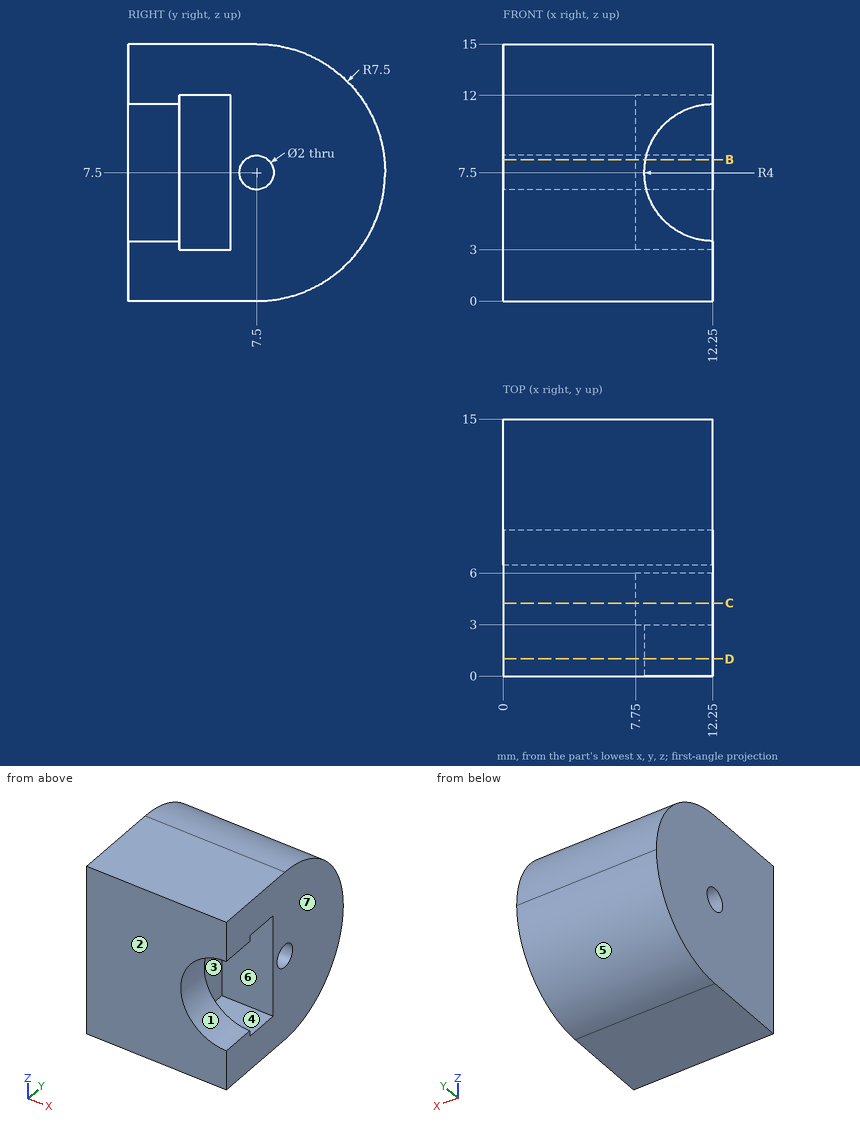
Can you work these out from the drawing? Everything is in mm from the part's minimum corner. A direction names the side the tool comes from. Coordinates: 2 decimals unless noted, no trailing zeros. Write each loop counter-clockwise with the first axis right and the second up, starting at its lowest first coordinate (ties: lowest second). Pieces come first, ordered by that corner, then holes. Notation, with made-up numbers: (-39.75, -25.75) -> (1.25, -25.75) arc R34 cw to (1.25, 13.25) -> close; hole circle Ø8 at (36, 0.5). An arc over 180 degrees is marked (long way). Return JSON: item names as keys, results as strings.
(1) Imagine slicing it at D-D, the plane y = 1. Please give me the cut outline in (x, z), then the cut area to 3 significant figures.
Numbers:
{"outline": "(0, 0) -> (12.25, 0) -> (12.25, 3.5) arc R4 cw to (12.25, 11.5) -> (12.25, 15) -> (0, 15) -> close", "area": "159 mm2"}
(2) We'd pull the mould along Y, two halves only. Please class the marked faces 4, 5, 6 and 7: +Y half, -Y half, draft (parallel to the pull), parting line (faces both ways), or undercut.
Numbers:
{"face 4": "undercut", "face 5": "+Y half", "face 6": "undercut", "face 7": "draft"}
(3) Imagine slicing it at C-C, the plane y = 4.25. Please give me the cut outline in (x, z), then the cut area to 3 significant figures.
Numbers:
{"outline": "(0, 0) -> (12.25, 0) -> (12.25, 3) -> (7.75, 3) -> (7.75, 12) -> (12.25, 12) -> (12.25, 15) -> (0, 15) -> close", "area": "143 mm2"}
(4) Imagine slicing it at B-B, the plane z = 8.25. Please give me the cut outline in (x, y), then the cut area to 3 significant figures.
Numbers:
{"outline": "(0, 0) -> (8.32, 0) -> (8.32, 3) -> (7.75, 3) -> (7.75, 6) -> (12.25, 6) -> (12.25, 6.84) -> (0, 6.84) -> close; (0, 8.16) -> (12.25, 8.16) -> (12.25, 14.96) -> (0, 14.96) -> close", "area": "142 mm2"}
(5) I'm going to push flat-ended pins straight in: pin 1 (3.5 mm diameter, centred on x = 9.5, z = 7, fed in from +Y); pin 2 (1.6 mm diameter, centred on y = 7.5, z = 7.5, fed in from +X); pin 3 (0.9 mm diameter, centred on y = 4.5, z = 6.5, fed in from +X); pin 4 (1.4 mm diameter, centred on x = 9.5, z = 8, fed in from -Y). Where does each tip first touch, or does it pass through?
Numbers:
{"pin 1": "stops at y = 15", "pin 2": "passes through", "pin 3": "stops at x = 7.75", "pin 4": "stops at y = 6"}
(6) I need wall thicknesses on L1, parallel to Z at x = 8, y = 7.5; L2, parallel to Y at x = 11, z = 8.25; L3, parallel to Y at x = 9, z = 3.75. Which ranges of each line are inside material? Lowest first, please.
Numbers:
{"L1": "z = 0 to 6.5, 8.5 to 15", "L2": "y = 6 to 6.84, 8.16 to 14.96", "L3": "y = 0 to 3, 6 to 14"}
(7) Which directions (+Z, -Z, +X, -X, +Y, -Y) give clear straight access to the entire face, cutting with the end or side of a thin tool? Please do the marked faces 1, 2 and 3.
Numbers:
{"face 1": "+X, -Y", "face 2": "+Z, -Z, +X, -X, -Y", "face 3": "+X"}
